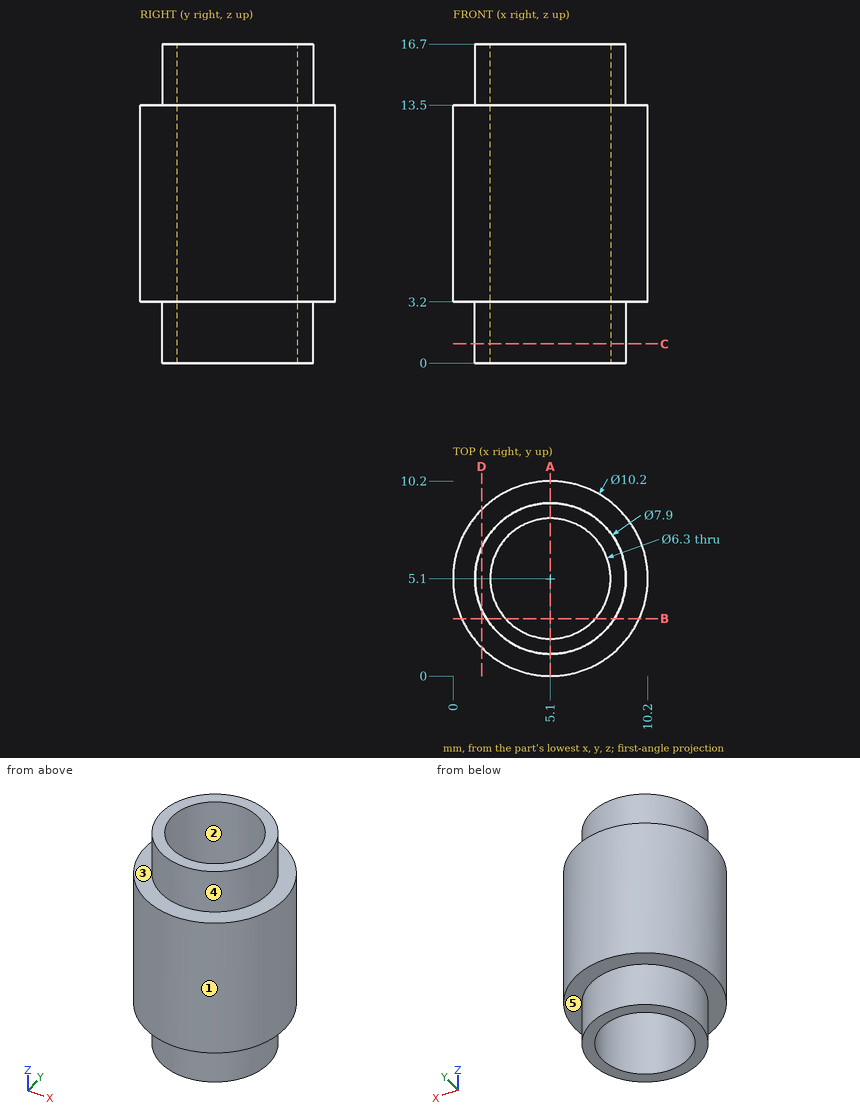
Can you work these out from the drawing? Everything is in mm from the part's minimum corner. A direction names the side the tool comes from. Round coordinates to 2 decimals unless told otherwise and drop trailing zeros. Write each loop counter-clockwise with the first axis right and the second up, starting at its lowest first coordinate (ties: lowest second). Pieces come first, ordered by that corner, then holes.
1. If we mould it in two halves opening along Y, with no side actions, what happens to the marked faces 1, 2 and 3? For each: released by +Y, released by -Y, zero draft, split by the parting line, or undercut.
2. Suppose I cut it at A-A (x = 5.1). List the corners of the cut face in (y, z) for me.
3. Will these pins go through, and if not, where does the flat tip stop? pin 1 Ø4 at (y, z) = (8, 9) entering from +X; pin 2 Ø1.5 at (x, z) = (2, 6) entering from -Y; pin 3 Ø6 at (y, z) = (8.5, 10.5) entering from +X.
4. Suppose I cut it at D-D (x = 1.5). List the corners of the cut face in (y, z) for me, and give its area (3 significant figures).
5. Suppose I cut it at B-B (y = 3). List the corners of the cut face in (x, z) for me, and give its area (3 significant figures).
6. I need wall thicknesses on L1, parallel to Y at x = 5.1, z = 10.5; L2, parallel to X at y = 5.75, z = 16.25. Which ranges of each line are inside material? Lowest first, please.
7. For the marked faces 4 and 5, which set-ups out of +Z, -Z, +X, -X, +Y, -Y let a thin tool reach every point of the face, with its end or its side?
8. Suppose I cut it at C-C (z = 1). List the corners of the cut face in (x, y) for me.
Answer sheet:
1. face 1: split by the parting line
1. face 2: undercut
1. face 3: zero draft
2. outline: (0, 3.2) - (1.15, 3.2) - (1.15, 0) - (1.95, 0) - (1.95, 16.7) - (1.15, 16.7) - (1.15, 13.5) - (0, 13.5) - close; (8.25, 0) - (9.05, 0) - (9.05, 3.2) - (10.2, 3.2) - (10.2, 13.5) - (9.05, 13.5) - (9.05, 16.7) - (8.25, 16.7) - close
3. pin 1: stops at x = 10.12
3. pin 2: stops at y = 0.57
3. pin 3: stops at x = 10.18
4. outline: (1.49, 3.2) - (3.47, 3.2) - (3.47, 0) - (6.73, 0) - (6.73, 3.2) - (8.71, 3.2) - (8.71, 13.5) - (6.73, 13.5) - (6.73, 16.7) - (3.47, 16.7) - (3.47, 13.5) - (1.49, 13.5) - close
4. area: 95.2 mm2
5. outline: (0.45, 3.2) - (1.75, 3.2) - (1.75, 0) - (2.75, 0) - (2.75, 16.7) - (1.75, 16.7) - (1.75, 13.5) - (0.45, 13.5) - close; (7.45, 0) - (8.45, 0) - (8.45, 3.2) - (9.75, 3.2) - (9.75, 13.5) - (8.45, 13.5) - (8.45, 16.7) - (7.45, 16.7) - close
5. area: 60.1 mm2
6. L1: y = 0 to 1.95, 8.25 to 10.2
6. L2: x = 1.2 to 2.02, 8.18 to 9
7. face 4: +Z
7. face 5: -Z
8. outline: circle Ø7.9 at (5.1, 5.1); hole circle Ø6.3 at (5.1, 5.1)
